Could you check a few things on this model? Use its own coordinates, in mm. Face numbers are marked on the shaded views. Give positions to 0.01 mm unless a question says otherwise; leave off trailing zeros. Order: outer loops, then holes, each group sorted by start corner. A loop starts at its lowest first (then second) coordinate and runs counter-clockwise, first axis right, second up. Notation, with made-up numbers: (67.5, -29) -> (80.5, -29) arc R25 cw to (80.5, -4) -> close; hole circle Ø3 at (-16, 8). An arc over 180 degrees is marked (long way). Answer as CSV lines item,"result". Start each with the question number.
(1) I want a section at C-C (z = 1.25). Please give me the cut outline in (x, y).
(2) I need wall thicknesses on L1, parallel to Y at x = -45, z = 6; L2, parallel to X at y = -8, z = 5; L3, parallel to X at y = 5, z = 7.25. Which ranges of each line are inside material? Lowest first, please.
(3) We'd pull the mould along Y, two halves only. Please class the marked faces 1, 2, 3 and 4: released by +Y, released by -Y, zero draft, split by the parting line, or undercut.
(4) Will this pin go through, and if not, where does the flat tip stop? pin 1 Ø4 at (x, y) = (43, -4.5) entering from -Z.
(5) I want a section at A-A (x = -45). Please give me the cut outline in (y, z), plus the area to 3 significant figures.
(6) I want a section at B-B (y = 0). Please give me the cut outline in (x, z).
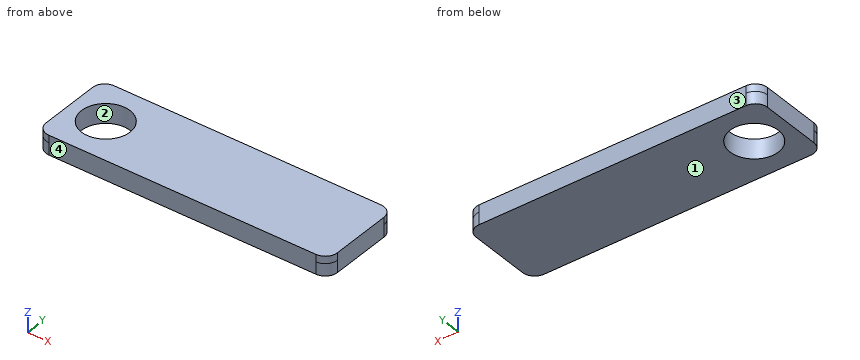
```python
from build123d import *

# Parameters (mm, degrees)
F0_W      = 120
F0_H      = 35
F0_R      = 10
F1_DEPTH  = 5
F2_R      = 5
F1_FACE_R = 10
F3_DEPTH  = 3


with BuildPart() as f1:
    # F0 (on Top) → F1 (new body)
    with BuildSketch(Plane.XY):
        Rectangle(F0_W, F0_H)
        with Locations((-45, 0)):
            Circle(F0_R, mode=Mode.SUBTRACT)
    extrude(amount=F1_DEPTH)

    # F2
    f2_edges = [f1.edges().sort_by_distance(p)[0] for p in [
        (-60, -17.5, 2.5),
        (-60, 17.5, 2.5),
        (60, 17.5, 2.5),
        (60, -17.5, 2.5),
    ]]
    fillet(f2_edges, radius=F2_R)

    # F1_face (on face) → F3 (join)
    with BuildSketch(Plane(origin=(3.658327, 0, 5), x_dir=(1, 0, 0), z_dir=(0, 0, 1))):
        with BuildLine():
            Line((-63.658327, 12.5), (-63.658327, -12.5))
            ThreePointArc((-63.658327, -12.5), (-62.193861, -16.035534), (-58.658327, -17.5))
            Line((-58.658327, -17.5), (51.341673, -17.5))
            ThreePointArc((51.341673, -17.5), (54.877207, -16.035534), (56.341673, -12.5))
            Line((56.341673, -12.5), (56.341673, 12.5))
            ThreePointArc((56.341673, 12.5), (54.877207, 16.035534), (51.341673, 17.5))
            Line((51.341673, 17.5), (-58.658327, 17.5))
            ThreePointArc((-58.658327, 17.5), (-62.193861, 16.035534), (-63.658327, 12.5))
        make_face()
        with Locations((-48.658327, 0)):
            Circle(F1_FACE_R, mode=Mode.SUBTRACT)
    extrude(amount=F3_DEPTH)


solid = f1.part
```
Final values:
1,outline,"(-60, -12.5) arc R5 ccw to (-55, -17.5) -> (55, -17.5) arc R5 ccw to (60, -12.5) -> (60, 12.5) arc R5 ccw to (55, 17.5) -> (-55, 17.5) arc R5 ccw to (-60, 12.5) -> close; hole circle Ø20 at (-45, 0)"
2,L1,"-17.5 to -10, 10 to 17.5"
2,L2,"-60 to -51, -39 to 60"
2,L3,"-60 to -53.66, -36.34 to 60"
3,face 1,"zero draft"
3,face 2,"undercut"
3,face 3,"released by +Y"
3,face 4,"released by -Y"
4,pin 1,"z = 0"
5,outline,"(-17.5, 0) -> (-10, 0) -> (-10, 8) -> (-17.5, 8) -> close; (10, 0) -> (17.5, 0) -> (17.5, 8) -> (10, 8) -> close"
5,area,"120 mm²"
6,outline,"(-60, 0) -> (-55, 0) -> (-55, 8) -> (-60, 8) -> close; (-35, 0) -> (60, 0) -> (60, 8) -> (-35, 8) -> close"
